```python
from build123d import *

# Parameters (mm, degrees)
F1_DEPTH  = 39.116
F2_DEPTH  = 9.144
F2_FACE_W = 84.796926
F2_FACE_H = 9.144
F3_DEPTH  = 21.59
F4_W      = 5.286065
F4_H      = 34.716484
F5_DEPTH  = 29.972
F7_DEPTH  = 49.784


with BuildPart() as f1:
    # F0 (on Top) → F1 (new body)
    with BuildSketch(Plane.XY):
        with BuildLine():
            ThreePointArc((29.291412, -4.666115), (-13.107051, 20.673092), (-55.505514, -4.666115))
            Line((-55.505514, -4.666115), (-55.505514, -9.459872))
            Line((-55.505514, -9.459872), (-43.261834, -9.459872))
            ThreePointArc((-43.261834, -9.459872), (-13.107051, 7.654781), (17.047732, -9.459872))
            Line((17.047732, -9.459872), (29.291412, -9.459872))
            Line((29.291412, -9.459872), (29.291412, -4.666115))
        make_face()
        with BuildLine():
            Line((-55.505514, -9.459872), (-55.505514, -4.666115))
            ThreePointArc((-55.505514, -4.666115), (-24.863895, -74.151052), (35.033861, -27.467821))
            ThreePointArc((35.033861, -27.467821), (33.57618, -15.710977), (29.291412, -4.666115))
            Line((29.291412, -4.666115), (29.291412, -9.459872))
            Line((29.291412, -9.459872), (17.047732, -9.459872))
            ThreePointArc((17.047732, -9.459872), (20.750825, -18.127512), (22.015551, -27.467821))
            ThreePointArc((22.015551, -27.467821), (-22.44736, -61.325697), (-43.261834, -9.459872))
            Line((-43.261834, -9.459872), (-55.505514, -9.459872))
        make_face()
    extrude(amount=F1_DEPTH)

    # F0 (on Top) → F2 (join)
    with BuildSketch(Plane.XY):
        with BuildLine():
            Line((29.291412, 70.322178), (-55.505514, 70.322178))
            Line((-55.505514, 70.322178), (-55.505514, -4.666115))
            ThreePointArc((-55.505514, -4.666115), (-13.107051, 20.673092), (29.291412, -4.666115))
            Line((29.291412, -4.666115), (29.291412, 70.322178))
        make_face()
    extrude(amount=F2_DEPTH)

    # F2_face (on face) → F3 (join)
    with BuildSketch(Plane(origin=(-13.107051, 70.322178, 4.572), x_dir=(-1, 0, 0), z_dir=(0, 1, 0))):
        Rectangle(F2_FACE_W, F2_FACE_H)
    extrude(amount=F3_DEPTH)

    # F4 (on face) → F5 (join)
    with BuildSketch(Plane.XY.offset(9.144)):
        with Locations((-12.872688, 37.945265)):
            Rectangle(F4_W, F4_H)
    extrude(amount=F5_DEPTH)

    # F6 (on face) → F7 (cut)
    with BuildSketch(Plane(origin=(-15.515721, 0, 0), x_dir=(0, -1, 0), z_dir=(-1, 0, 0))):
        Polygon((-55.303507, 9.144), (-20.612797, 39.116), (-55.303507, 39.116), align=None)
    extrude(amount=-F7_DEPTH, mode=Mode.SUBTRACT)


solid = f1.part
```
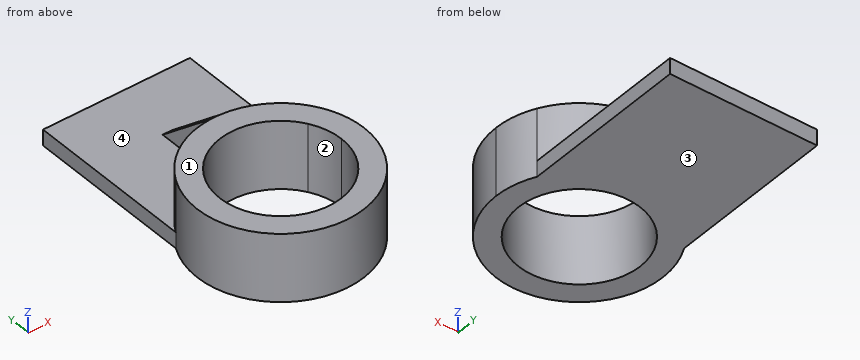
Design review of the part built by this model. Coordinates are the model's own, in mm. Face numbers are marked on the shaded views. A direction names the side the tool comes from. Coordinates: 2 decimals unless noted, no trailing zeros. Order: outer loops, then holes, each group sorted by start corner. A loop starts at its lowest first (then second) coordinate and runs counter-clockwise, first axis right, second up.
1) Mouldability with a two-part tool opening along X and no side actions: class the marked faces 1 and 2 as +X half, -X half, draft (parallel to the pull), parting line (faces both ways), or undercut.
2) Take a section at A-A, the plane z = 4.5. Give the boundary of the cut face in (x, y).
3) Take a section at D-D, the plane y = 22.5. Give the boundary of the cut face in (x, z).
4) Take a section at B-B, the plane x = 1.5. Give the boundary of the cut face in (y, z).
5) For the marked faces 3 and 4, list the 3-axis set-ups (+Z, -Z, +X, -X, +Y, -Y) from which the entire face can be reached by the end or side of a thin tool; tool diameter is ignored.
6) Wall thickness on line 1 along Z through (x, y) = (29, 17.5); line 2 along X through (y, z) = (-56, 26); line 3 along Y through (x, z) = (-6, 19): over which ranges is each line inside the solid? List them lowest first.
7) Take a section at C-C, the plane y = 0. Give the boundary of the cut face in (x, z).
8) Clearance check with flat-ended pins moving along their axes: pin 1 (4 mm diameter, centred on y = -52.5, z = 19.5, fed in from +X); pin 2 (7.5 mm diameter, centred on y = 64, z = 6, fed in from -X); pin 3 (12 mm diameter, centred on x = 5.5, z = 4.5, fed in from -Y). State where each tip first meets the part, or that it passes through.
Returned:
1. face 1: draft
1. face 2: undercut
2. outline: (-55.51, -4.67) arc R48.14 ccw (long way) to (35.03, -27.47) arc R48.14 ccw to (29.29, -4.67) - (29.29, 91.91) - (-55.51, 91.91) - close; hole (17.05, -9.46) arc R35.12 ccw (long way) to (22.02, -27.47) arc R35.12 ccw to start
3. outline: (-55.51, 0) - (29.29, 0) - (29.29, 9.14) - (-10.23, 9.14) - (-10.23, 37.49) - (-15.52, 37.49) - (-15.52, 9.14) - (-55.51, 9.14) - close
4. outline: (-73.34, 0) - (-59.41, 0) - (-59.41, 39.12) - (-73.34, 39.12) - close; (4.47, 0) - (91.91, 0) - (91.91, 9.14) - (18.4, 9.14) - (18.4, 39.12) - (4.47, 39.12) - close
5. face 3: -Z, +X, -X, +Y, -Y
5. face 4: +Z, +Y
6. line 1: z = 0 to 9.14
6. line 2: x = -51.88 to -33.59, 7.37 to 25.67
6. line 3: y = -75.08 to -61.86, 6.93 to 20.15
7. outline: (-55.51, 0) - (-35, 0) - (-35, 39.12) - (-52.64, 39.12) - (-52.64, 9.14) - (-55.51, 9.14) - close; (8.78, 0) - (29.29, 0) - (29.29, 9.14) - (26.43, 9.14) - (26.43, 39.12) - (8.78, 39.12) - close
8. pin 1: stops at x = 29.17
8. pin 2: stops at x = -55.51
8. pin 3: stops at y = -73.93
